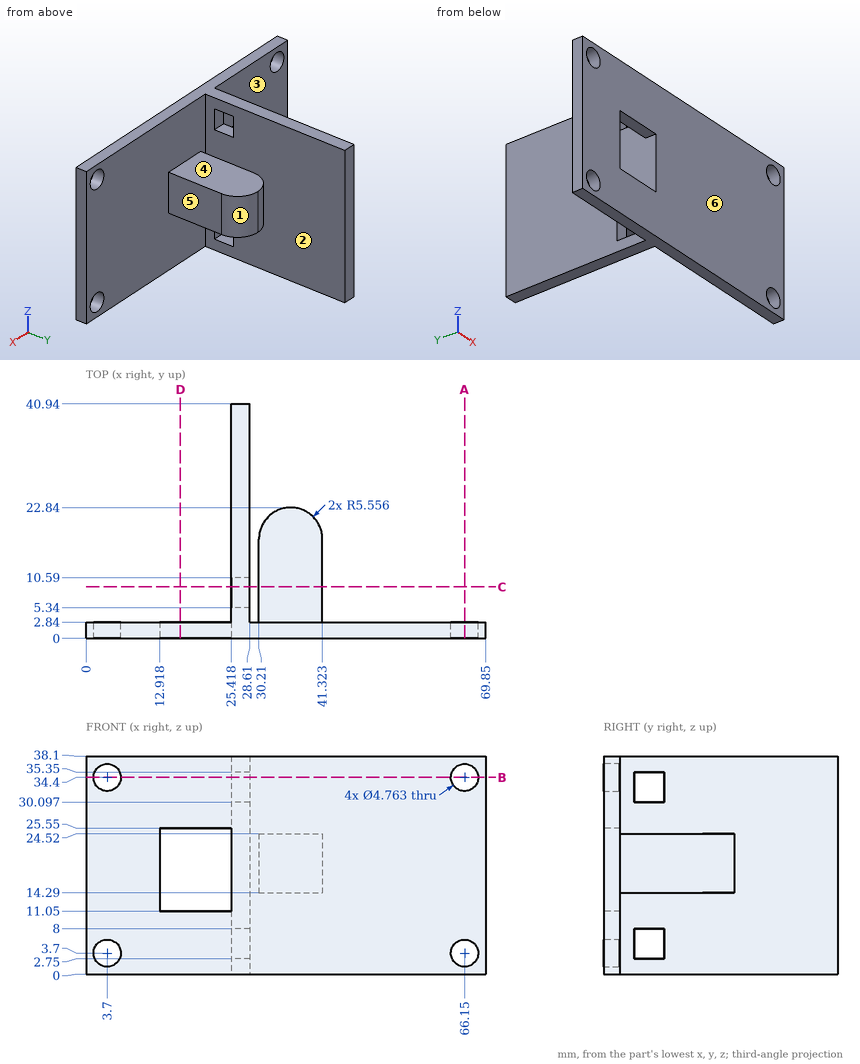
Print and shaded views of the part. All mm, measured from the part's lowest x, y and z. A direction names the side the tool comes from. Give positions to 0.01 mm unless a question says otherwise; leave off trailing zeros. Order: outer loops, then holes, each group sorted by start corner. A loop starts at its lowest first (then second) coordinate and runs counter-clockwise, first axis right, second up. Notation, with made-up numbers: (75, 26) -> (126, 26) arc R32 cw to (126, 63) -> close; hole circle Ø1 at (13.5, 52). An arc over 180 degrees is marked (long way). Use CSV: the item, a comma, the result in double quotes.
1. Band-saw the part on D-D, the plane x = 16.5. Give the cut face in (y, z).
Outcome:
outline,"(0, 0) -> (2.84, 0) -> (2.84, 11.05) -> (0, 11.05) -> close; (0, 25.55) -> (2.84, 25.55) -> (2.84, 38.1) -> (0, 38.1) -> close"
2. Drop flat-ended pins along their axis: pin 1 (10 mm diameter, centred on y = 12.5, z = 26.5, fed in from +X); pin 2 (9 mm diameter, centred on x = 36, y = 15, fed in from -Z); pin 3 (12.5 mm diameter, centred on x = 9.5, z = 20, fed in from +Y). Give the stop position or say it passes through.
Outcome:
pin 1,"x = 41.32"
pin 2,"z = 14.29"
pin 3,"y = 2.84"
3. Drill centre lines: line 1 along X through (y, z) = (1, 34.4); line 2 along Z through (x, y) = (66.15, 1.4); line 3 along X through (y, z) = (1, 34). Where is each one in solid material? Low to high. Write a range as from..to.
Outcome:
line 1,"0..1.32, 6.08..63.77, 68.53..69.85"
line 2,"0..1.32, 6.08..32.02, 36.78..38.1"
line 3,"0..1.35, 6.05..63.8, 68.5..69.85"
4. Band-saw the part on C-C, the plane y = 9. Give the cut face in (x, z).
Outcome:
outline,"(25.42, 0) -> (28.61, 0) -> (28.61, 2.75) -> (25.42, 2.75) -> close; (25.42, 8) -> (28.61, 8) -> (28.61, 30.1) -> (25.42, 30.1) -> close; (25.42, 35.35) -> (28.61, 35.35) -> (28.61, 38.1) -> (25.42, 38.1) -> close; (30.21, 14.29) -> (41.32, 14.29) -> (41.32, 24.52) -> (30.21, 24.52) -> close"
5. Band-saw the part on A-A, the plane x = 66.15. Give the cut face in (y, z).
Outcome:
outline,"(0, 0) -> (2.84, 0) -> (2.84, 1.32) -> (0, 1.32) -> close; (0, 6.08) -> (2.84, 6.08) -> (2.84, 32.02) -> (0, 32.02) -> close; (0, 36.78) -> (2.84, 36.78) -> (2.84, 38.1) -> (0, 38.1) -> close"
6. 3-axis set-ups, long thin cutter, end or side, ignore diameter. For the marked faces 4, 5 and 6: which of +Z, -Z, +X, -X, +Y, -Y reach the whole face in a straight line?
Outcome:
face 4,"+Z, +X, +Y"
face 5,"+Z, -Z, +X, +Y"
face 6,"+Z, -Z, +X, -X, -Y"
7. Mould opens along X. For the marked faces 1, 2 and 3 say: +X half, -X half, draft (parallel to the pull), parting line (faces both ways), or undercut.
Outcome:
face 1,"+X half"
face 2,"undercut"
face 3,"draft"
8. Band-saw the part on B-B, the plane z = 34.4. Give the cut face in (x, y), then the cut area to 3 significant figures.
Outcome:
outline,"(0, 0) -> (1.32, 0) -> (1.32, 2.84) -> (0, 2.84) -> close; (6.08, 0) -> (63.77, 0) -> (63.77, 2.84) -> (28.61, 2.84) -> (28.61, 5.34) -> (25.42, 5.34) -> (25.42, 2.84) -> (6.08, 2.84) -> close; (25.42, 10.59) -> (28.61, 10.59) -> (28.61, 40.94) -> (25.42, 40.94) -> close; (68.53, 0) -> (69.85, 0) -> (69.85, 2.84) -> (68.53, 2.84) -> close"
area,"276 mm²"
